Verification items for the finished model (mm, model axes). Face numbers are marked on the shaded views. A direction names the side the tool comes from. Coordinates: 2 decimals unless noted, no trailing zeros. Order: outer loops, then holes, each group sorted by start corner. A loop starts at its lowest first (then second) coordinate and runs counter-clockwise, first axis right, second up. Notation, with made-up numbers: M -19,87 L 18,87 A33 ccw 18,115 Z; hole C 5.5,-18.5 d2. An arc over 180 degrees is marked long. Return JSON: item names as keys, results as strings. Group by question number.
Q1. Mould release check, pull along Z, two halves, no side actions. Record for the marked faces 5, 6, 7 and 8: pulls with the +Z half, pulls with the -Z half, needs draft (parallel to the pull), parting line crosses it, or undercut.
Q2. Section check C-C, the plane y = -14. Count the separate pieces of the cut face and the enclosed holes in it, then the cut area to 3 significant figures.
Q3. Section check B-B, the plane y = -28. Enter the section's corners in (x, z), then the cut area to 3 significant figures.
Q4. Access from +Z, -Z, +X, -X, +Y, -Y to the whole of each face (thin tool, end or side, straight path). Record for the marked faces 1, 2, 3 and 4.
Q5. Section check A-A, the plane z = -9. Enter the section's corners in (x, y), then the cut area to 3 significant figures.
Q6. Go/stop test with flat-tipped pins: pin 1 Ø10 at (y, z) = (-24, -18.5) entering from -X; pin 2 Ø7.5 at (x, y) = (51, -17) entering from +Z; pin 3 Ø17 at (y, z) = (-15.5, -12) entering from +X. Record where each tip stops, or that it passes through.
Q7. Thickness scan on probe 1 along X at (y, z) = (-8.5, -16); probe 2 along Z at (x, y) = (21, -17); probe 3 along Y at (x, z) = (-45, -58.5). Record the ranges inside material, lowest first.
Q8. Section check D-D, the plane x = -27. Enter the section's corners in (y, z), then the cut area to 3 significant figures.
from build123d import *

# Parameters (mm, degrees)
F1_DEPTH = 34
F2_R     = 6
F3_DEPTH = 90.001
F4_R     = 5
F5_DEPTH = 67.22541
F7_DEPTH = 67.22541


with BuildPart() as f1:
    # F0 (on Front) → F1 (new body)
    with BuildSketch(Plane.XZ):
        Polygon((-12.5, -2.22441), (-32.5, -2.22441), (-32.5, -55.22441), (-57.5, -55.22441), (-57.5, -67.22441), (-11.515748, -67.22441), (-11.515748, -52.22441), (0, -52.22441), (11.515748, -52.22441), (11.515748, -67.22441), (57.5, -67.22441), (57.5, -55.22441), (32.5, -55.22441), (32.5, -2.22441), (12.5, -2.22441), (12.5, -40.22441), (0, -40.22441), (-12.5, -40.22441), align=None)
    extrude(amount=F1_DEPTH)

    # F2 (on face) → F3 (cut, through all)
    with BuildSketch(Plane.YZ.offset(32.5)):
        with Locations((-17, -22.22441)):
            Circle(F2_R)
    extrude(amount=-F3_DEPTH, mode=Mode.SUBTRACT)

    # F4 (on Top) → F5 (cut, through all)
    with BuildSketch(Plane.XY):
        with Locations((-45, -12)):
            Circle(F4_R)
        with Locations((45, -12)):
            Circle(F4_R)
    extrude(amount=-F5_DEPTH, mode=Mode.SUBTRACT)

    # F6 (on Top) → F7 (cut, through all)
    with BuildSketch(Plane.XY):
        Polygon((57.5, -34), (57.5, -22), (45.5, -34), align=None)
        Polygon((-45.5, -34), (-57.5, -22), (-57.5, -34), align=None)
    extrude(amount=-F7_DEPTH, mode=Mode.SUBTRACT)


solid = f1.part
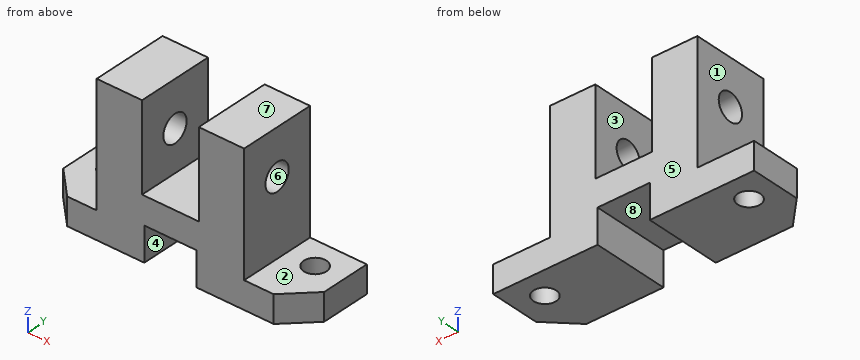
Numbers:
{
 "1": {"face 5": "needs draft", "face 6": "undercut", "face 7": "pulls with the +Z half", "face 8": "pulls with the -Z half"},
 "2": {"separate pieces": "5", "enclosed holes": "0", "area": "2,890 mm2"},
 "3": {"outline": "M -51.5,-67.22 L -11.52,-67.22 L -11.52,-52.22 L 11.52,-52.22 L 11.52,-67.22 L 51.5,-67.22 L 51.5,-55.22 L 32.5,-55.22 L 32.5,-2.22 L 12.5,-2.22 L 12.5,-40.22 L -12.5,-40.22 L -12.5,-2.22 L -32.5,-2.22 L -32.5,-55.22 L -51.5,-55.22 Z", "area": "3,390 mm2"},
 "4": {"face 1": "+Z, -X, +Y, -Y", "face 2": "+Z, +X, +Y, -Y", "face 3": "+Z, +Y, -Y", "face 4": "-Z, +Y, -Y"},
 "5": {"outline": "M -32.5,-34 L -12.5,-34 L -12.5,0 L -32.5,0 Z; M 12.5,-34 L 32.5,-34 L 32.5,0 L 12.5,0 Z", "area": "1,360 mm2"},
 "6": {"pin 1": "stops at x = -32.5", "pin 2": "stops at z = -55.22", "pin 3": "stops at x = 32.5"},
 "7": {"probe 1": "x = -32.5 to -12.5, 12.5 to 32.5", "probe 2": "z = -67.22 to -28.22, -16.22 to -2.22", "probe 3": "y = -34 to -17, -7 to 0"},
 "8": {"outline": "M -34,-67.22 L 0,-67.22 L 0,-2.22 L -34,-2.22 Z; hole C -17,-22.22 d12", "area": "2,100 mm2"}
}
